The listing builds one solid part. Answer for the finished solid, in the listing's coordinates (mm). Face numbers are marked on the shaded views. A direction names the side the tool comes from. Round coordinates to 2 decimals unless told otherwise and drop trailing zeros. Write each loop counter-clockwise with the first axis right and the second up, starting at its lowest first coordinate (ties: lowest second). Pieces come first, ordered by that corner, then holes. Notation, with made-up numbers: (48, 18.25) - (93, 18.25) arc R19 cw to (93, 41.25) - close; hole circle Ø5 at (84, 29.25). An arc over 180 degrees is marked (long way). Return JSON: item names as keys, results as strings. Group by question number.
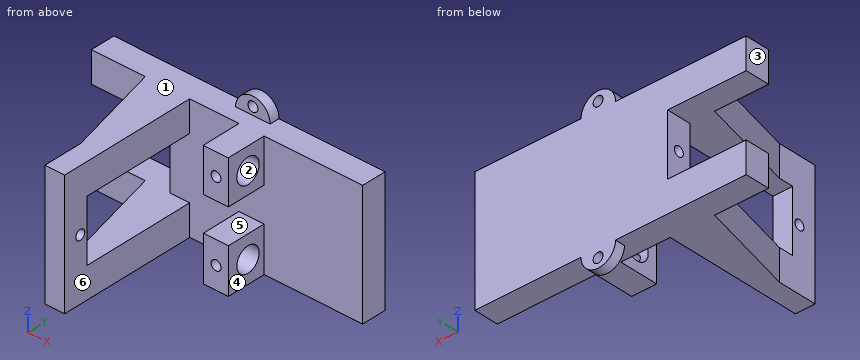
from build123d import *

# Parameters (mm, degrees)
F0_W          = 55
F0_H          = 25
F1_DEPTH      = 5
F2_W          = 15.9233940393
F2_H          = 12.5
F3_DEPTH      = 5.001
F4_R          = 1
F5_DEPTH      = 3.5
F7_DEPTH      = 28
F8_W          = 23
F8_H          = 12.5
F9_DEPTH      = 39.0776059607
F10_R         = 1
F11_DEPTH     = 39.0776059607
F12_W         = 5.0766059607
F12_H         = 8.8610539977
F12_H_2       = 9.1389460023
F13_DEPTH     = 8
F14_R         = 2.5
F15_DEPTH     = 10
F16_T1_DEPTH  = 6.25
F16_T3_DEPTH  = 6.25
F16_T8_DEPTH  = 58.1925499954
F16_T14_DEPTH = 58.1925499954
F17_R         = 1
F18_DEPTH     = 3
F20_DEPTH     = 2
F21_R         = 1
F22_DEPTH     = 2.001


# Not quite as in the source:
# - a fillet or chamfer that OpenCascade refuses, or shapes differently, is made with other operations: its cross-section is extruded or revolved along the edge and cut away or added


with BuildPart() as f1:
    # F0 (on Front) → F1 (new body)
    with BuildSketch(Plane.XZ):
        Rectangle(F0_W, F0_H)
    extrude(amount=F1_DEPTH)

    # F2 (on face) → F3 (cut, through all)
    with BuildSketch(Plane.XZ.offset(5)):
        with Locations((-19.5383029804, 0)):
            Rectangle(F2_W, F2_H)
    extrude(amount=-F3_DEPTH, mode=Mode.SUBTRACT)

    # F4 (on face) → F5 (cut)
    with BuildSketch(Plane(origin=(-11.5766059607, 0, 0), x_dir=(0, -1, 0), z_dir=(-1, 0, 0))):
        with Locations((2.5, 0)):
            Circle(F4_R)
    extrude(amount=-F5_DEPTH, mode=Mode.SUBTRACT)

    # F6 (on face) → F7 (join)
    with BuildSketch(Plane.XZ.offset(5)):
        Polygon((-7.5766059607, 12.5), (-11.5766059607, 12.5), (-11.5766059607, 6.25), (-11.5766059607, -6.25), (-11.5766059607, -12.5), (-7.5766059607, -12.5), align=None)
    extrude(amount=F7_DEPTH)

    # F8 (on face) → F9 (cut, through all)
    with BuildSketch(Plane(origin=(-11.5766059607, 0, 0), x_dir=(0, -1, 0), z_dir=(-1, 0, 0))):
        with Locations((16.5, 0)):
            Rectangle(F8_W, F8_H)
    extrude(amount=-F9_DEPTH, mode=Mode.SUBTRACT)

    # F10 (on face) → F11 (cut, through all)
    with BuildSketch(Plane(origin=(-11.5766059607, 0, 0), x_dir=(0, -1, 0), z_dir=(-1, 0, 0))):
        with Locations((29.5, 0)):
            Circle(F10_R)
    extrude(amount=-F11_DEPTH, mode=Mode.SUBTRACT)

    # F12 (on face) → F13 (join)
    with BuildSketch(Plane.XZ.offset(5)):
        with Locations((4.9616970196, 8.0694730012)):
            Rectangle(F12_W, F12_H)
        with Locations((4.9616970196, -7.9305269988)):
            Rectangle(F12_W, F12_H_2)
    extrude(amount=F13_DEPTH)

    # F14 (on face) → F15 (cut)
    with BuildSketch(Plane.YZ.offset(7.5)):
        with Locations((-8.6, 8)):
            Circle(F14_R)
        with Locations((-8.6, -8)):
            Circle(F14_R)
    extrude(amount=-F15_DEPTH, mode=Mode.SUBTRACT)

    # F16: chamfer of 20 x 5 on 2 edges, made by hand

    # F16_s2 → F16_t1 (join)
    with BuildSketch(Plane.XY.offset(6.25)):
        Polygon((-11.5766059607, -25), (-16.5766059607, -5), (-11.5766059607, -5), align=None)
    extrude(amount=F16_T1_DEPTH)

    # F16_s4 → F16_t3 (join)
    with BuildSketch(Plane.XY.offset(-12.5)):
        Polygon((-11.5766059607, -25), (-16.5766059607, -5), (-11.5766059607, -5), align=None)
    extrude(amount=F16_T3_DEPTH)


with BuildPart() as f16_tool6:
    # F16_s7 → F16_t8 (new body)
    with BuildSketch(Plane.XY.offset(12.5)):
        Polygon((-11.5766059607, -25), (-16.5766059607, -5), (-11.5766059607, -5), align=None)
    extrude(amount=-F16_T8_DEPTH)

    split(bisect_by=Plane.XY.offset(-6.25), keep=Keep.BOTTOM)

    split(bisect_by=Plane.XY.offset(-12.5), keep=Keep.TOP)


with BuildPart() as f1_1:
    add(f1.part)

    # F16_t5: union F16_tool6
    add(f16_tool6.part)


with BuildPart() as f16_tool12:
    # F16_s13 → F16_t14 (new body)
    with BuildSketch(Plane.XY.offset(45.6925499954)):
        Polygon((-11.5766059607, -25), (-16.5766059607, -5), (-11.5766059607, -5), align=None)
    extrude(amount=-F16_T14_DEPTH)

    split(bisect_by=Plane.XY.offset(12.5), keep=Keep.BOTTOM)

    split(bisect_by=Plane.XY.offset(6.25), keep=Keep.TOP)


with BuildPart() as f1_2:
    add(f1_1.part)

    # F16_t11: union F16_tool12
    add(f16_tool12.part)

    # F17 (on face) → F18 (cut)
    with BuildSketch(Plane.XZ.offset(13)):
        with Locations((5, 8)):
            Circle(F17_R)
        with Locations((5, -8)):
            Circle(F17_R)
    extrude(amount=-F18_DEPTH, mode=Mode.SUBTRACT)

    # F19 (on face) → F20 (join)
    with BuildSketch(Plane(origin=(0, 0, 0), x_dir=(-1, 0, 0), z_dir=(0, 1, 0))):
        with BuildLine():
            Line((1, -12.5), (-6, -12.5))
            ThreePointArc((-6, -12.5), (-2.5, -16), (1, -12.5))
        make_face()
        with BuildLine():
            Line((-6, 12.5), (1, 12.5))
            ThreePointArc((1, 12.5), (-2.5, 16), (-6, 12.5))
        make_face()
    extrude(amount=-F20_DEPTH)

    # F21 (on face) → F22 (cut, through all)
    with BuildSketch(Plane.XZ.offset(2)):
        with Locations((2.5334937964, 14.1)):
            Circle(F21_R)
        with Locations((2.5334937964, -14.1)):
            Circle(F21_R)
    extrude(amount=-F22_DEPTH, mode=Mode.SUBTRACT)


solid = f1_2.part
(1) Find section A-A (z = -8). Write down the section's boundary in (x, y).
(2) Find section D-D (z = 11.5). Write down the section's boundary in (x, y).
(3) Flat-ended cylindrical pins translate along their axes: pin 1 (10 mm diameter, centred on x = -6, y = -14.5, fed in from +Z); pin 2 (3 mm diameter, centred on y = -28, z = 2, fed in from -X); pin 3 (5.5 mm diameter, centred on x = 5, z = 9.5, fed in from -Y); pin 4 (1.6 mm diameter, centred on y = -29.5, z = 0, fed in from +X). Find the tip coordinate at first contact, or state that the pin passes through.
(4) Determine the mould class of the marked faces 1, 2 and 3 for opening direction Z: +Z half, -Z half, draft (parallel to the pull), parting line (faces both ways), or undercut.
(5) Consider line 1 (X direction, y = -12.4, z = -8); line 2 (Z direction, x = -10.3, y = -29.5); line 3 (Z direction, x = 3, y = -8). Determine where each line is inside the solid, lowest interval first.
(6) Find section B-B (y = -29.5). Write down the section's boundary in (x, z).
(7) Find section C-C (x = -10.5). Write down the section's boundary in (y, z).
(8) For the marked faces 4, 5 and 6, determine the directions among +Z, -Z, +X, -X, +Y, -Y from which every point of the face is accessible in a straight line to the end or side of a thin tool.
Check sheet entries:
{
 "1": {"outline": "(-27.5, -5) - (-16.58, -5) - (-11.58, -25) - (-11.58, -33) - (-7.58, -33) - (-7.58, -5) - (2.42, -5) - (2.42, -6.1) - (7.5, -6.1) - (7.5, -5) - (27.5, -5) - (27.5, 0) - (-27.5, 0) - close; (2.42, -13) - (4, -13) - (4, -11.1) - (2.42, -11.1) - close; (6, -13) - (7.5, -13) - (7.5, -11.1) - (6, -11.1) - close"},
 "2": {"outline": "(-27.5, -5) - (-16.58, -5) - (-11.58, -25) - (-11.58, -33) - (-7.58, -33) - (-7.58, -5) - (2.42, -5) - (2.42, -13) - (7.5, -13) - (7.5, -5) - (27.5, -5) - (27.5, 0) - (-27.5, 0) - close"},
 "3": {"pin 1": "stops at z = 12.5", "pin 2": "stops at x = -11.58", "pin 3": "stops at y = -13", "pin 4": "passes through"},
 "4": {"face 1": "+Z half", "face 2": "undercut", "face 3": "draft"},
 "5": {"line 1": "x = -14.73 to -7.58, 2.42 to 4, 6 to 7.5", "line 2": "z = -12.5 to -1, 1 to 12.5", "line 3": "z = -12.5 to -10.43, -5.57 to -3.36, 3.64 to 5.57, 10.43 to 12.5"},
 "6": {"outline": "(-11.58, -12.5) - (-7.58, -12.5) - (-7.58, -1) - (-11.58, -1) - close; (-11.58, 1) - (-7.58, 1) - (-7.58, 12.5) - (-11.58, 12.5) - close"},
 "7": {"outline": "(-33, -12.5) - (0, -12.5) - (0, 12.5) - (-33, 12.5) - close; hole circle Ø2 at (-29.5, 0); hole (-28, -6.25) - (-5, -6.25) - (-5, 6.25) - (-28, 6.25) - close; hole circle Ø2 at (-2.5, 0)"},
 "8": {"face 4": "+Z, -Z, +X, -Y", "face 5": "+X, -X, -Y", "face 6": "+Z, -Z, -Y"}
}
